Source: CAD feature listing. Evaluate the final solid. Frame: model axes, mm. Face numbers are marked on the shaded views. A direction names the side the tool comes from. Round coordinates to 2 decimals unless told otherwise and drop trailing zeros. Order: outer loops, then holes, each group sorted by start corner. A loop starts at its lowest first (then second) coordinate and runs counter-clockwise, first axis right, second up. Notation, with made-up numbers: (72, 79) -> (126, 79) arc R31 ccw to (126, 106) -> close; hole circle Ø8 at (77, -14). An arc over 180 degrees is marked (long way). Write item = value, one per line. Start each with the question number.
(1) Contact query for flat-ended pins moving along their axis: pin 1 Ø2 at (y, z) = (38, -0.5) entering from +X; pin 2 Ø6 at (y, z) = (12, -19.5) entering from +X; pin 3 Ø19 at (x, z) = (69, 1) entering from +Y. Output: stop coordinate, or through.
(2) Cut plane D-D on y = 20. Return the cut outline in (x, z).
(3) Reachability of the marked faces 5, 6, 7, 8 and 9 from +Z, -Z, +X, -X, +Y, -Y: full face, straight path, thin tool, end or side. Return the list, or none.
(4) Cut plane C-C on z = -24. Return the cut outline in (x, y).
(5) Cut plane A-A on y = 9. Return the cut outline in (x, z), then the cut area to 3 significant figures.
(6) Ray query, line 1 (X direction, y = 45, z = -21); line 2 (X direction, y = 16.5, z = 28); line 3 (Y direction, x = 77, z = -11.5). Return the intervals inside material, ascending.
(7) Draft query along Z for the marked faces 1, 2, 3 and 4. Return one class per face: released by +Z, released by -Z, zero draft, split by the parting line, or undercut.
(8) Cut plane B-B on x = 74. Return the cut outline in (y, z).
Autodesk Fusion 360 part; units mm, degrees
sketch "Sketch1" plane through (0, 0, 0) normal (0, 0, 1) x (1, 0, 0)
  line L0 (0, 0) -> (88, 0)
  line L1 (88, 0) -> (88, 24)
  line L2 (88, 24) -> (76, 24)
  line L3 (76, 24) -> (76, 56)
  line L4 (76, 56) -> (0, 56)
  line L5 (0, 56) -> (0, 0)
  dimension "d1" = 88
  dimension "d2" = 24
  dimension "d3" = 12
  dimension "d4" = 32
extrude "Extrude1" add sketch "Sketch1" along normal mid plane 64
sketch "Sketch2" plane through (0, 0, 0) normal (0, 0, 1) x (1, 0, 0)
  line L0 (88, 0) -> (108, 0)
  line L1 (108, 0) -> (94, 24)
  line L2 (94, 24) -> (88, 24)
  line L3 (88, 24) -> (88, 0)
  point P0 (88, 24)
  point P1 (88, 0)
  dimension "d7" = 20
  dimension "d8" = 6
extrude "Extrude2" add sketch "Sketch2" along normal mid plane 24
sketch "Sketch3" plane through (0, 56, 0) normal (0, 1, 0) x (-1, 0, 0)
  line L0 (0, -32) -> (0, 32)
  line L1 (0, 32) -> (-76, 32)
  line L2 (-76, 32) -> (-76, -32)
  line L3 (-76, -32) -> (0, -32)
  circle A0 centre (-76, 0) radius 20
  dimension "d11" = 40
extrude "Extrude3" cut sketch "Sketch3" against normal blind 32 contours L2 A0 picked at (-67.9161, 5.5729)
sketch "Sketch4" plane through (0, 0, 0) normal (-1, 0, 0) x (0, 0, 1)
  line L0 (-32, 0) -> (32, 0)
  line L1 (32, 0) -> (32, 56)
  line L2 (32, 56) -> (-32, 56)
  line L3 (-32, 56) -> (-32, 0)
  circle A0 centre (32, 56) radius 44
  dimension "d14" = 88
extrude "Extrude4" cut sketch "Sketch4" against normal blind 44 contours L1 L2 A0 picked at (29.9127, 26.816)
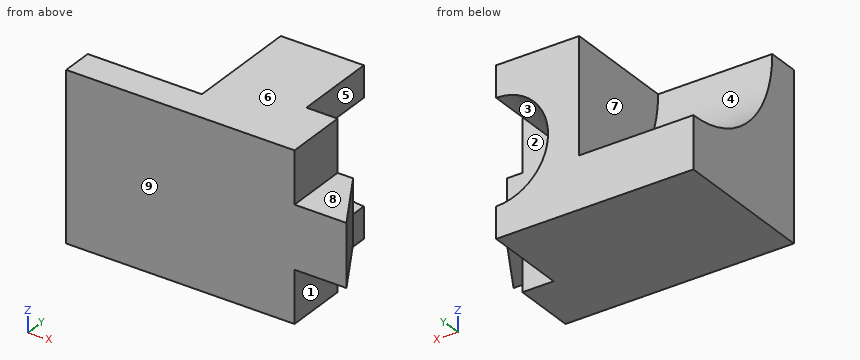
Evaluation:
q1.pin_1 = 56.06
q1.pin_2 = 88
q1.pin_3 = 24
q2.outline = (0, -32) -> (88, -32) -> (88, -12) -> (96.33, -12) -> (96.33, 12) -> (88, 12) -> (88, 32) -> (44, 32) -> (44, 6.7) -> (0, 6.7) -> close
q3.face_5 = +Z, -Z, +X, +Y
q3.face_6 = +Z, +X, -X, +Y, -Y
q3.face_7 = +Z, -X, +Y
q3.face_8 = +Z, +X, +Y, -Y
q3.face_9 = +Z, -Z, +X, -X, -Y
q4.outline = (0, 0) -> (88, 0) -> (88, 24) -> (76, 24) -> (76, 56) -> (0, 56) -> close
q5.outline = (0, -32) -> (88, -32) -> (88, -12) -> (102.75, -12) -> (102.75, 12) -> (88, 12) -> (88, 32) -> (0, 32) -> close
q5.area = 5,990 mm^2
q6.line_1 = 0 to 76
q6.line_2 = 44 to 88
q6.line_3 = 0 to 24
q7.face_1 = zero draft
q7.face_2 = undercut
q7.face_3 = undercut
q7.face_4 = released by +Z
q8.outline = (0, -32) -> (56, -32) -> (56, -19.9) -> (24, -19.9) -> (24, 19.9) -> (56, 19.9) -> (56, 32) -> (0, 32) -> close
